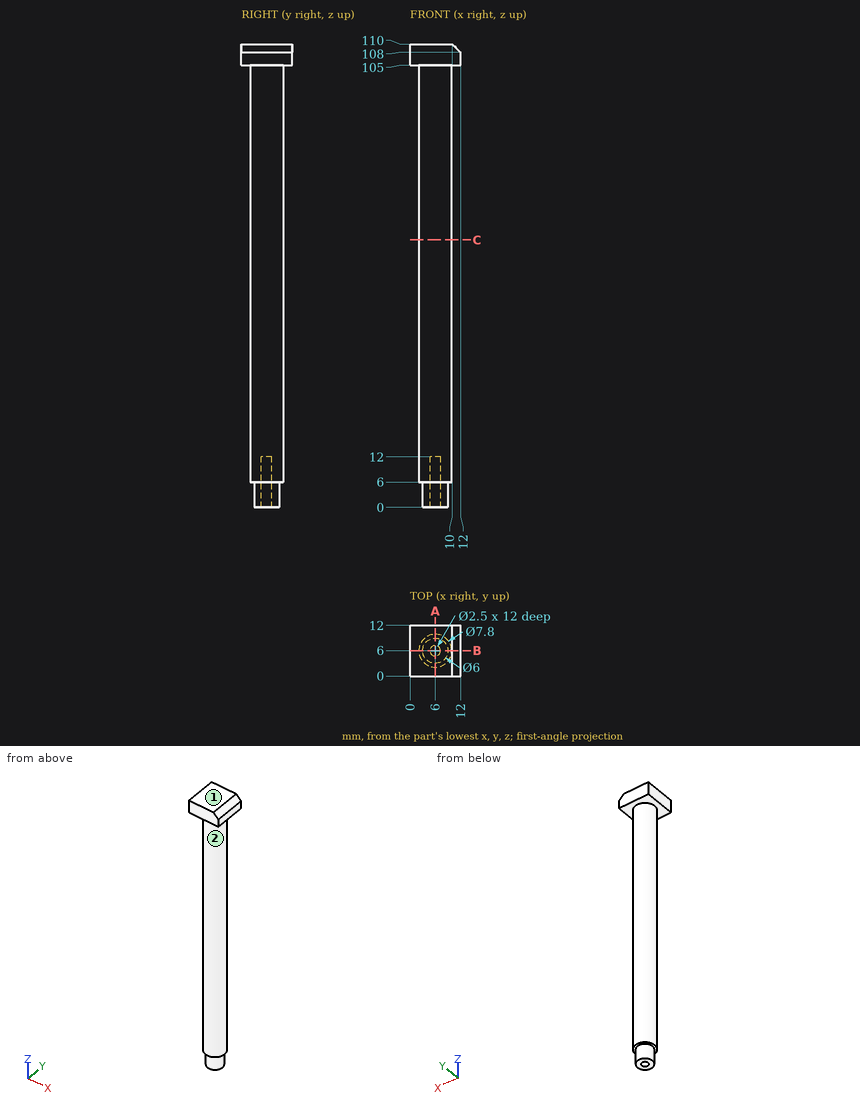
Design review of the part shown in the three views and the two pictorial views. Dimensions are in mm from the part's minimum x, y and z. A direction names the side the tool comes from. Give positions to 0.01 mm unless a question says otherwise; leave off trailing zeros. Order: outer loops, then holes, each group sorted by start corner. A loop starts at its lowest first (then second) coordinate and runs counter-clockwise, first axis right, second up. Notation, with made-up numbers: M 10.25,-21.5 L 55.25,-21.5 A8 ccw 55.25,-14.5 Z; hole C -33.5,-12.75 d6. An arc over 180 degrees is marked long. Answer in a Markdown table with one row per item. Add a question column.
(1) Consider section A-A on x = 6. State the section outline as (y, z) points.
(2) Consider section C-C on z = 63.5. State the section outline as (x, y) points, and give its area (3 significant figures).
(3) For the marked faces 1 and 2, list the 3-axis set-ups (+Z, -Z, +X, -X, +Y, -Y) from which the entire face can be reached by the end or side of a thin tool; tool diameter is ignored.
(4) For pin 1 (6 mm diameter, centred on y = 4.5, z = 67.5, fed in from -X); pin 2 (1.5 mm diameter, centred on x = 5.5, y = 9, fed in from -Z); pin 3 (5 mm diameter, centred on y = 2, z = 59.5, fed in from +X); pin 4 (1 mm diameter, centred on y = 3, z = 55, fed in from -X), all flat-tipped, find the tip position at first contact; note any pin that passes through.
(5) Wall thickness on probe 1 along Y at (x, z) = (6, 8.5); probe 2 along Y at (x, z) = (6, 5); probe 3 along X at (y, z) = (8.5, 61): over which ranges is each line inside the solid? List them lowest first. Write a range as [from, to].
(6) Consider section B-B on y = 6. State the section outline as (x, z) points.
Evaluation:
| question | item | result |
|---|---|---|
| 1 | outline | M 0,105 L 2.1,105 L 2.1,6 L 3,6 L 3,0 L 4.75,0 L 4.75,12 L 7.25,12 L 7.25,0 L 9,0 L 9,6 L 9.9,6 L 9.9,105 L 12,105 L 12,110 L 0,110 Z |
| 2 | outline | C 6,6 d7.8 |
| 2 | area | 47.8 mm^2 |
| 3 | face 1 | +Z, +X, -X, +Y, -Y |
| 3 | face 2 | -Z |
| 4 | pin 1 | stops at x = 2.1 |
| 4 | pin 2 | stops at z = 0 |
| 4 | pin 3 | stops at x = 9.6 |
| 4 | pin 4 | stops at x = 3.01 |
| 5 | probe 1 | y = [2.1, 4.75], [7.25, 9.9] |
| 5 | probe 2 | y = [3, 4.75], [7.25, 9] |
| 5 | probe 3 | x = [3.01, 8.99] |
| 6 | outline | M 0,105 L 2.1,105 L 2.1,6 L 3,6 L 3,0 L 4.75,0 L 4.75,12 L 7.25,12 L 7.25,0 L 9,0 L 9,6 L 9.9,6 L 9.9,105 L 12,105 L 12,108 L 10,110 L 0,110 Z |
